from build123d import *

# Parameters (mm, degrees)
SKETCH1_W           = 30
SKETCH1_H           = 65
SKETCH1_R           = 1.375
BOSS_EXTRUDE1_DEPTH = 0.8
SKETCH4_R           = 3
SKETCH4_R_2         = 1.375
EXTRUDE_THIN1_DEPTH = 0.1
FILLET1_R           = 3
SKETCH2_W           = 12.5
SKETCH2_H           = 16
BOSS_EXTRUDE2_DEPTH = 1.6
SKETCH3_W           = 5
SKETCH3_H           = 50.8
BOSS_EXTRUDE3_DEPTH = 2.54
SKETCH5_W           = 5.5
SKETCH5_H           = 8
BOSS_EXTRUDE4_DEPTH = 2


with BuildPart() as part:
    # Sketch1 → Boss-Extrude1 (new, symmetric)
    with BuildSketch(Plane.XY):
        Rectangle(SKETCH1_W, SKETCH1_H)
        with Locations((11.5, -29)):
            Circle(SKETCH1_R, mode=Mode.SUBTRACT)
        with Locations((-11.5, -29)):
            Circle(SKETCH1_R, mode=Mode.SUBTRACT)
        with Locations((11.5, 29)):
            Circle(SKETCH1_R, mode=Mode.SUBTRACT)
        with Locations((-11.5, 29)):
            Circle(SKETCH1_R, mode=Mode.SUBTRACT)
    extrude(amount=BOSS_EXTRUDE1_DEPTH, both=True)

    # Sketch4 → Extrude-Thin1 (add)
    # profile 1 of 4: a face of its own
    with BuildSketch(Plane.XY.offset(0.8)):
        with Locations((11.5, 29)):
            Circle(SKETCH4_R)
        with Locations((11.5, 29)):
            Circle(SKETCH4_R_2, mode=Mode.SUBTRACT)
    # profile 2 of 4: a face of its own
    with BuildSketch(Plane.XY.offset(0.8)):
        with Locations((11.5, -29)):
            Circle(SKETCH4_R)
        with Locations((11.5, -29)):
            Circle(SKETCH4_R_2, mode=Mode.SUBTRACT)
    # profile 3 of 4: a face of its own
    with BuildSketch(Plane.XY.offset(0.8)):
        with Locations((-11.5, -29)):
            Circle(SKETCH4_R)
        with Locations((-11.5, -29)):
            Circle(SKETCH4_R_2, mode=Mode.SUBTRACT)
    # profile 4 of 4: a face of its own
    with BuildSketch(Plane.XY.offset(0.8)):
        with Locations((-11.5, 29)):
            Circle(SKETCH4_R)
        with Locations((-11.5, 29)):
            Circle(SKETCH4_R_2, mode=Mode.SUBTRACT)
    extrude(amount=EXTRUDE_THIN1_DEPTH)

    # Fillet1
    fillet1_edges = [part.edges().sort_by_distance(p)[0] for p in [
        (-15, -32.5, 0),
        (-15, 32.5, 0),
        (15, 32.5, 0),
        (15, -32.5, 0),
    ]]
    fillet(fillet1_edges, radius=FILLET1_R)

    # Sketch2 → Boss-Extrude2 (add)
    with BuildSketch(Plane.XY.offset(0.8)):
        with Locations((1.9, 27.5)):
            Rectangle(SKETCH2_W, SKETCH2_H)
    extrude(amount=BOSS_EXTRUDE2_DEPTH)

    # Sketch3 → Boss-Extrude3 (add)
    with BuildSketch(Plane.XY.offset(0.8)):
        with Locations((11.5, 0)):
            Rectangle(SKETCH3_W, SKETCH3_H)
    extrude(amount=BOSS_EXTRUDE3_DEPTH)

    # Sketch5 → Boss-Extrude4 (add)
    with BuildSketch(Plane.XY.offset(0.8)):
        with Locations((-13.25, -21.5)):
            Rectangle(SKETCH5_W, SKETCH5_H)
        with Locations((-13.25, -8.9)):
            Rectangle(SKETCH5_W, SKETCH5_H)
    extrude(amount=BOSS_EXTRUDE4_DEPTH)


solid = part.part
Read the model definition and answer for the solid it produces. Units are mm, in the model's axes. A direction names the side the tool comes from. Coordinates: 2 decimals unless noted, no trailing zeros. Loops run counter-clockwise (first coordinate to the right, second up) from the corner with the lowest first, then second, coordinate; pieces in that order, holes last. Notation, with made-up numbers: (-14.5, -28.75) -> (44.5, -28.75) arc R28 cw to (44.5, -4.75) -> close; hole circle Ø2 at (8, 9.25). An arc over 180 degrees is marked (long way). Write item = value, one per line. Start each with the question number.
1) The part is cut by section C-C, the plane x = -5. Determine the outline of the cut face in (y, z).
2) For faces 1 (the face through (2, 28, 2.4)), 2 (the face through (13, 28, 0.9)), 3 (the face through (13, -30, 0.9)), 4 (the face through (-15, 0, 0)), determine the directions among +Z, -Z, +X, -X, +Y, -Y from which every point of the face is accessible in a straight line to the end or side of a thin tool.
3) The part is cut by section B-B, the plane x = 2.5. Determine the outline of the cut face in (y, z), plus the area to 3 significant figures.
4) Given P1, Ø0.8, axis at x = -15.5, y = -10.5, coming from the -Z side; P2, Ø5, axis at x = 11, y = 29, coming from the +Z side; P3, Ø1.6, axis at x = -13, z = 2, coming from the -Y side; P4, Ø3, axis at x = 11.5, y = -29, coming from the -Z side, each flat-ended and moving along its own axis, determine where each tip first touches the part or whether it passes through.
5) The part is cut by section A-A, the plane y = -11. Determine the outline of the cut face in (x, z), plus the area to 3 significant figures.
6) Find the intervals of material crossed by L1, parallel to Y at x = 11.5, z = 0.2 (3 decimals); L2, parallel to Y at x = -15, z = 1.4; L3, parallel to X at y = 23, z = 0.9, in increasing order. Write a range as from..to.
7) The mould has two halves that part along X. Classify faces 5 (the face through (14.14, -31.6, 0.01)), 6 (the face through (2, 34, 0.8)), 7 (the face through (11.321, -27.637, 0.038)): pulls with the +X half, pulls with the -X half, needs draft (parallel to the pull), parting line crosses it, or undercut.
Result:
q1.outline = (-32.5, -0.8) -> (32.5, -0.8) -> (32.5, 0.8) -> (-32.5, 0.8) -> close
q2.face_1 = +Z, -X, +Y, -Y
q2.face_2 = +Z, +X, +Y
q2.face_3 = +Z, +X, -X, -Y
q2.face_4 = -Z, -X, +Y, -Y
q3.outline = (-32.5, -0.8) -> (32.5, -0.8) -> (32.5, 0.8) -> (35.5, 0.8) -> (35.5, 2.4) -> (19.5, 2.4) -> (19.5, 0.8) -> (-32.5, 0.8) -> close
q3.area = 130 mm²
q4.P1 = 0.8
q4.P2 = 0.9
q4.P3 = -25.5
q4.P4 = -0.8
q5.outline = (-16, 0.8) -> (-15, 0.8) -> (-15, -0.8) -> (15, -0.8) -> (15, 0.8) -> (14, 0.8) -> (14, 3.34) -> (9, 3.34) -> (9, 0.8) -> (-10.5, 0.8) -> (-10.5, 2.8) -> (-16, 2.8) -> close
q5.area = 71.7 mm²
q6.L1 = -32.5..-30.375, -27.625..27.625, 30.375..32.5
q6.L2 = -25.5..-17.5, -12.9..-4.9
q6.L3 = -4.35..8.15, 9..14
q7.face_5 = pulls with the +X half
q7.face_6 = needs draft
q7.face_7 = undercut
